from build123d import *

# Parameters (mm, degrees)
SKETCH_1_R            = 38
EXTRUDE_1_DEPTH       = 39
SKETCH_3_R            = 17.5
EXTRUDE_2_DEPTH       = 7
SKETCH_5_R            = 12
CUT_EXTRUDE_2_DEPTH   = 46
CHAMFER_2_SIZE        = 1
CHAMFER_2_SIZE2       = 0.577350269
SKETCH_6_R            = 12.5
SKETCH_6_R_2          = 12
EXTRUDE_4_DEPTH       = 1
SKETCH_7_R            = 16
SKETCH_7_R_2          = 13
CUT_EXTRUDE_5_DEPTH   = 2
FILLET_5_R            = 1
CUT_EXTRUDE_12_DEPTH  = 2
EXTRUDE_START         = 30
EXTRUDE_7_DEPTH       = 24
SKETCH_16_R           = 6.5
SKETCH_16_R_2         = 6
EXTRUDE_9_DEPTH       = 6
SKETCH_17_R           = 0.5
EXTRUDE_10_DEPTH      = 5
SKETCH_18_R           = 12.5
CUT_EXTRUDE_13_DEPTH  = 86.164546614
SKETCH_19_R           = 17.5
CUT_EXTRUDE_14_DEPTH  = 7
HOLE_WIZARD_M51_D     = 5.8
HOLE_WIZARD_M51_DEPTH = 14
HOLE_WIZARD_M51_TIP   = 1.742495795


with BuildPart() as part:
    # Эскиз1 → Бобышка-Вытянуть1 (new body)
    with BuildSketch(Plane.XY):
        Circle(SKETCH_1_R)
    extrude(amount=EXTRUDE_1_DEPTH)

    # Эскиз3 → Бобышка-Вытянуть2 (add)
    with BuildSketch(Plane.XY.offset(39)):
        Circle(SKETCH_3_R)
    extrude(amount=EXTRUDE_2_DEPTH)

    # Эскиз5 → Вырез-Вытянуть2 (cut)
    with BuildSketch(Plane.XY.offset(46)):
        Circle(SKETCH_5_R)
    extrude(amount=-CUT_EXTRUDE_2_DEPTH, mode=Mode.SUBTRACT)

    # Фаска2
    chamfer_2_edges = [part.edges().sort_by_distance(p)[0] for p in [
        (-12, 0, 46),
    ]]
    chamfer_2_side = [part.faces().sort_by_distance(p)[0] for p in [
        (-17.005025253, 0, 46),
    ]]
    chamfer(chamfer_2_edges, length=CHAMFER_2_SIZE, length2=CHAMFER_2_SIZE2, reference=chamfer_2_side[0])

    # Эскиз6 → Бобышка-Вытянуть4 (add)
    with BuildSketch(Plane(origin=(0, 0, 0), x_dir=(-1, 0, 0), z_dir=(0, 0, -1))):
        with Locations(Location((0, 0, 0), (0, 0, 180))):
            Circle(SKETCH_6_R)
        with Locations(Location((0, 0, 0), (0, 0, 180))):
            Circle(SKETCH_6_R_2, mode=Mode.SUBTRACT)
    extrude(amount=EXTRUDE_4_DEPTH)

    # Эскиз7 → Вырез-Вытянуть5 (cut)
    with BuildSketch(Plane(origin=(0, 0, 0), x_dir=(-1, 0, 0), z_dir=(0, 0, -1))):
        Circle(SKETCH_7_R)
        Circle(SKETCH_7_R_2, mode=Mode.SUBTRACT)
    extrude(amount=-CUT_EXTRUDE_5_DEPTH, mode=Mode.SUBTRACT)

    # Скругление5
    fillet_5_edges = [part.edges().sort_by_distance(p)[0] for p in [
        (16, 0, 0),
    ]]
    fillet(fillet_5_edges, radius=FILLET_5_R)

    # Эскиз8 → Вырез-Вытянуть12 (cut)
    with BuildSketch(Plane.XY.offset(39)):
        with BuildLine():
            Line((17.98928511, 4.316899492), (17.840599274, -4.895203525))
            ThreePointArc((17.840599274, -4.895203525), (-0.298556122, -18.497590769), (-17.98928511, -4.316899492))
            Line((-17.98928511, -4.316899492), (-17.840599274, 4.895203525))
            ThreePointArc((-17.840599274, 4.895203525), (0.298556122, 18.497590769), (17.98928511, 4.316899492))
        make_face()
    extrude(amount=-CUT_EXTRUDE_12_DEPTH, mode=Mode.SUBTRACT)


with BuildPart() as cut_extrude_12_piece_1:
    # of the separate pieces the step leaves, piece 1, a body of its own (cut_extrude_12_pieces)
    add(part.part.solids().sort_by_distance((-17, 0, 0))[0])

    # Эскиз10 → Бобышка-Вытянуть7 (add)
    with BuildSketch(Plane(origin=(0, 0, 0), x_dir=(1, 0, 0), z_dir=(0, 1, 0)).offset(EXTRUDE_START)):
        Polygon((-12.104871286, -25.970188702), (11.895058188, -26.028371648), (11.953241134, -2.028442174), (-12.04668834, -1.970259229), align=None)
    extrude(amount=EXTRUDE_7_DEPTH)

    # Эскиз16 → Бобышка-Вытянуть9 (add)
    with BuildSketch(Plane(origin=(0, 54, 0), x_dir=(1, 0, 0), z_dir=(0, 1, 0))):
        with Locations(Location((0, -14.052210171, 0), (0, 0, 90))):
            Circle(SKETCH_16_R)
        with Locations(Location((0, -14.052210171, 0), (0, 0, 270))):
            Circle(SKETCH_16_R_2, mode=Mode.SUBTRACT)
    extrude(amount=EXTRUDE_9_DEPTH)

    # Эскиз17 → Бобышка-Вытянуть10 (add)
    with BuildSketch(Plane(origin=(0, 54, 0), x_dir=(1, 0, 0), z_dir=(0, 1, 0))):
        with Locations(Location((-3.512245794, -12.5530062, 0), (0, 0, 90))):
            Circle(SKETCH_17_R)
        with Locations(Location((0.020111582, -12.538765356, 0), (0, 0, 90))):
            Circle(SKETCH_17_R)
        with Locations(Location((3.508572113, -12.538765356, 0), (0, 0, 90))):
            Circle(SKETCH_17_R)
        with Locations(Location((3.471979869, -15.527131894, 0), (0, 0, 90))):
            Circle(SKETCH_17_R)
        with Locations(Location((-0.016480661, -15.588118967, 0), (0, 0, 90))):
            Circle(SKETCH_17_R)
        with Locations(Location((-3.529336021, -15.551526723, 0), (0, 0, 90))):
            Circle(SKETCH_17_R)
        with Locations(Location((-1.746429893, -11.03259915, 0), (0, 0, 90))):
            Circle(SKETCH_17_R)
        with Locations(Location((1.76817255, -10.974982716, 0), (0, 0, 90))):
            Circle(SKETCH_17_R)
        with Locations(Location((1.782576658, -17.082324667, 0), (0, 0, 90))):
            Circle(SKETCH_17_R)
        with Locations(Location((-1.804046327, -17.125536992, 0), (0, 0, 90))):
            Circle(SKETCH_17_R)
    extrude(amount=EXTRUDE_10_DEPTH)


with BuildPart() as cut_extrude_12_piece_2:
    # of the separate pieces the step leaves, piece 2, a body of its own (cut_extrude_12_pieces)
    add(part.part.solids().sort_by_distance((17.5, 0, 39))[0])


with BuildPart() as cut_extrude_13_tool:
    # Эскиз18 → Вырез-Вытянуть13 (new, through all)
    with BuildSketch(Plane(origin=(0, 0, -1), x_dir=(-1, 0, 0), z_dir=(0, 0, -1))):
        with Locations(Location((0, 0, 0), (0, 0, 180))):
            Circle(SKETCH_18_R)
    extrude(amount=-CUT_EXTRUDE_13_DEPTH)


with BuildPart() as cut_extrude_12_piece_1_1:
    add(cut_extrude_12_piece_1.part)

    # Вырез-Вытянуть13: cut by cut_extrude_13_tool
    add(cut_extrude_13_tool.part, mode=Mode.SUBTRACT)

    # Отверстие с зазором M51
    with Locations(Plane(origin=(-26.772593493, 3.813867052, 39), x_dir=(1, 0, 0), z_dir=(0, 0, 1))):
        with Locations((0, 0), (0, -7.627734104), (53.545186986, 0), (53.545186986, -7.627734104)):
            Hole(HOLE_WIZARD_M51_D / 2, depth=HOLE_WIZARD_M51_DEPTH)
            with Locations((0, 0, -(HOLE_WIZARD_M51_DEPTH + HOLE_WIZARD_M51_TIP / 2))):  # 118° drill point
                Cone(0, HOLE_WIZARD_M51_D / 2, HOLE_WIZARD_M51_TIP, mode=Mode.SUBTRACT)


with BuildPart() as cut_extrude_12_piece_2_1:
    add(cut_extrude_12_piece_2.part)

    # Вырез-Вытянуть13: cut by cut_extrude_13_tool
    add(cut_extrude_13_tool.part, mode=Mode.SUBTRACT)

    # Эскиз19 → Вырез-Вытянуть14 (cut)
    with BuildSketch(Plane.XY.offset(46)):
        Circle(SKETCH_19_R)
    extrude(amount=-CUT_EXTRUDE_14_DEPTH, mode=Mode.SUBTRACT)


solid = cut_extrude_12_piece_1_1.part
Part model, mm, in its own coordinate system. A direction names the side the tool comes from. Coordinates: 2 decimals unless noted, no trailing zeros. Order: outer loops, then holes, each group sorted by start corner. A loop starts at its lowest first (then second) coordinate and runs counter-clockwise, first axis right, second up.
(1) Slice it at A-A, the plane z = 35.5. Write the cut outline in (x, y), and give its area (3 significant figures).
Check sheet entries:
outline: circle Ø76 at (0, 0); hole circle Ø5.8 at (-26.77, -3.81); hole circle Ø5.8 at (-26.77, 3.81); hole circle Ø25 at (0, 0); hole circle Ø5.8 at (26.77, -3.81); hole circle Ø5.8 at (26.77, 3.81)
area: 3,940 mm2
(2) Pin check, flat tips, straight feed: pin 1 Ø10 at (x, z) = (6, 27.5) entering from -Y; pin 2 Ø0.8 at (x, z) = (1.5, 17) entering from +Y; pin 3 Ø10 at (x, z) = (-25.5, 21) entering from -Y. Stop position of each tip, or through.
Check sheet entries:
pin 1: stops at y = -37.99
pin 2: stops at y = 59
pin 3: stops at y = -32
(3) Tool access for faces 4 (the face through (0.264, 56.958, 8.058)), 5 (the face through (10.316, -7.91, 0.986)), 6 (the face through (0, 18.5, 38)): list every direction of +Z, -Z, +X, -X, +Y, -Y with a clear straight run to the whole face (end or side of a thin tool).
Check sheet entries:
face 4: +Y
face 5: -Z
face 6: +Z
(4) Pull direction X, two halves, no side cores. Call faces 1 (the face through (0, -18.5, 38)), 2 (the face through (2.49, 56.96, 8.05)), 3 (the face through (-6.8, 10.7, 0)): pulls with the +X half, pulls with the -X half, needs draft (parallel to the pull), parting line crosses it, or undercut.
Check sheet entries:
face 1: undercut
face 2: parting line crosses it
face 3: needs draft
(5) Slice it at B-B, the plane z = 5. Write the cut outline in (x, y), and give its area (3 significant figures).
Check sheet entries:
outline: (-12.05, 36.04) arc R38 ccw (long way) to (11.95, 36.07) - (11.95, 54) - (-12.05, 54) - close; hole circle Ø25 at (0, 0)
area: 4,440 mm2
(6) Slice it at C-C, the plane x = 20. Write the cut outline in (y, z).
Check sheet entries:
outline: (-32.31, 0) - (32.31, 0) - (32.31, 39) - (-32.31, 39) - close
(7) Probe L1, parallel to Y at x = 0, z = 1; L2, parallel to Y at x = 0, z = 16; L3, parallel to X at y = 49, z = 10. List the from-to ranges inside material, lowest first.
Check sheet entries:
L1: y = -38 to -16, -13 to -12.5, 12.5 to 13, 16 to 38
L2: y = -38 to -12.5, 12.5 to 59
L3: x = -12.07 to 11.93
